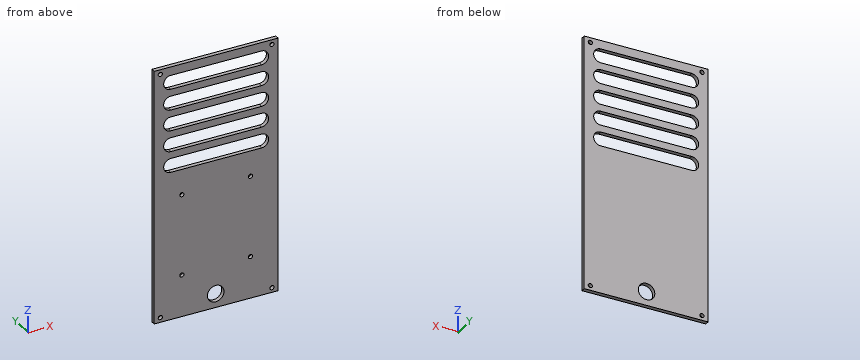
Autodesk Inventor part; units mm, degrees
ref_plane "YZ Plane" through (0, 0, 0) normal (1, 0, 0) x (0, 1, 0)
ref_plane "XZ Plane" through (0, 0, 0) normal (0, 1, 0) x (-1, 0, 0)
ref_plane "XY Plane" through (0, 0, 0) normal (0, 0, 1) x (1, 0, 0)
sketch "Skizze1" plane through (0, 0, 0) normal (0, 1, 0) x (-1, 0, 0)
  line L0 (-44.3, 91.2) -> (44.3, 91.2)
  line L1 (44.3, 91.2) -> (44.3, -91.2)
  line L2 (44.3, -91.2) -> (-44.3, -91.2)
  line L3 (-44.3, -91.2) -> (-44.3, 91.2)
  line L4 (-44.3, 91.2) -> (44.3, -91.2) construction
  line L5 (44.3, 91.2) -> (-44.3, -91.2) construction
  point P0 (0, 0)
  dimension "d0" = 88.6
  dimension "d1" = 182.4
extrude "Extrusion1" add sketch "Skizze1" along normal blind 3
sketch "Skizze2" plane through (0, 0, 0) normal (0, -1, 0) x (1, 0, 0)
  line L0 (-44.3, -91.2) -> (44.3, -91.2)
  line L1 (0, -91.2) -> (0, 91.2)
  line L2 (44.3, 91.2) -> (-44.3, 91.2)
  line L3 (-24.5, -61.2) -> (24.5, -61.2)
  line L4 (24.5, -61.2) -> (24.5, -3.2)
  line L5 (24.5, -3.2) -> (-24.5, -3.2)
  line L6 (-24.5, -3.2) -> (-24.5, -61.2)
  line L7 (-24.5, -61.2) -> (24.5, -3.2) construction
  line L8 (24.5, -61.2) -> (-24.5, -3.2) construction
  point P0 (0, 0)
  point P1 (0, -32.2)
  dimension "d5" = 49
  dimension "d6" = 58
  dimension "d7" = 30
hole "Bohrung1" at (-24.5, 0, -61.2) at (24.5, 0, -61.2) at (24.5, 0, -3.2) at (-24.5, 0, -3.2) direction (0, 1, 0) diameter 3 depth 2.5
sketch "Skizze3" plane through (0, 0, 0) normal (0, -1, 0) x (1, 0, 0)
  line L0 (32.5, 15.0873) -> (-32.5, 15.0873)
  line L1 (-37.5, 20.0873) -> (-37.5, 20.0873)
  line L2 (-32.5, 25.0873) -> (32.5, 25.0873)
  line L3 (37.5, 20.0873) -> (37.5, 20.0873)
  line L4 (37.5, 15.0873) -> (-37.5, 25.0873) construction
  line L5 (-37.5, 15.0873) -> (37.5, 25.0873) construction
  arc A0 (-37.5, 20.0873) -> (-32.5, 15.0873) centre (-32.5, 20.0873) ccw
  arc A1 (-32.5, 25.0873) -> (-37.5, 20.0873) centre (-32.5, 20.0873) ccw
  arc A2 (32.5, 15.0873) -> (37.5, 20.0873) centre (32.5, 20.0873) ccw
  arc A3 (37.5, 20.0873) -> (32.5, 25.0873) centre (32.5, 20.0873) ccw
  point P0 (0, 0)
  point P1 (0, 20.0873)
  dimension "d15" = 75
  dimension "d16" = 10
  dimension "d18" = 5
  dimension "d19" = 5
  dimension "d20" = 5
extrude "Extrusion2" cut sketch "Skizze3" against normal blind 10
pattern_linear "Rechteckige Anordnung1" count 5 spacing 15 along (0, 0, 1) of "Extrusion2"
hole "Bohrung2" at (-39.9, 0, -87.8) direction (0, 1, 0) diameter 3 depth 8 tip angle 118
mirror "Spiegeln1" about plane through (0, 0, 0) normal (1, 0, 0) of "Bohrung2"
mirror "Spiegeln2" about plane through (0, 0, 0) normal (0, 0, 1) of "Bohrung2", "Spiegeln1"
hole "Bohrung3" at (-0.3, 0, -81.2) direction (0, 1, 0) diameter 11.8 depth 8 tip angle 118
properties part number "RaspberryBox_Backplate_v2"
Input: part model. Units: mm. Frame: model coordinates. Give positions to 0.01 mm unless a question says otherwise; leave off trailing zeros. Loops run counter-clockwise (first coordinate to the right, second up) from the corner with the lowest first, then second, coordinate; pieces in that order, holes last.
1) Section query D-D on z = 17. Return the cut outline in (x, y).
A:
outline: (-44.3, 0) - (-36.43, 0) - (-36.43, 3) - (-44.3, 3) - close; (36.43, 0) - (44.3, 0) - (44.3, 3) - (36.43, 3) - close
2) Line query: L1, parallel to X at y = 0.6, z = -3.2; L2, parallel to Z at x = 31.5, y = 2.6; L3, parallel to X at y = 1, z = 87.8. Output: solid intervals per line, ascending.
A:
L1: x = -44.3 to -26, -23 to 23, 26 to 44.3
L2: z = -91.2 to 15.09, 25.09 to 30.09, 40.09 to 45.09, 55.09 to 60.09, 70.09 to 75.09, 85.09 to 91.2
L3: x = -44.3 to -41.4, -38.4 to 38.4, 41.4 to 44.3
3) Section query C-C on y = 0.6. Count the separate pieces of the cut face and the enclosed holes in it, and give its area (3 significant figures).
A:
separate pieces: 1
enclosed holes: 14
area: 12,400 mm2
4) Section query B-B on x = -20. Return the cut outline in (y, z), and give its area (3 significant figures).
A:
outline: (0, -91.2) - (3, -91.2) - (3, 15.09) - (0, 15.09) - close; (0, 25.09) - (3, 25.09) - (3, 30.09) - (0, 30.09) - close; (0, 40.09) - (3, 40.09) - (3, 45.09) - (0, 45.09) - close; (0, 55.09) - (3, 55.09) - (3, 60.09) - (0, 60.09) - close; (0, 70.09) - (3, 70.09) - (3, 75.09) - (0, 75.09) - close; (0, 85.09) - (3, 85.09) - (3, 91.2) - (0, 91.2) - close
area: 397 mm2
5) Contact query for a flat-ended pin moving along its axis: pin 1 (2.5 mm diameter, centred on x = 24.5, z = -61, fed in from -Y). Output: stop coordinate, or through.
A:
pin 1: stops at y = 2.5
6) Section query A-A on z = -81.2. Return the cut outline in (x, y), and give its area (3 significant figures).
A:
outline: (-44.3, 0) - (-6.2, 0) - (-6.2, 3) - (-44.3, 3) - close; (5.6, 0) - (44.3, 0) - (44.3, 3) - (5.6, 3) - close
area: 230 mm2
